The listing builds one solid part. Answer for the finished solid, in the listing's coordinates (mm). A direction names the side the tool comes from. Coordinates: 2 decimals unless noted, no trailing zeros. Order: outer loops, then holes, each group sorted by start corner. A loop starts at its lowest first (then second) coordinate and runs counter-clockwise, first axis right, second up. Notation, with made-up numbers: (-31, 64.5) -> (3, 64.5) arc R26 ccw to (3, 90.5) -> close; hole circle Ø11 at (43, -30). An arc over 180 degrees is marked (long way). Write each question's results on one line, items separated by ' | '. Start each with the question number.
(1) The part is cut by section B-B, the plane z = 37.5. Give the vertices of the cut face in (x, y), then the cut area to 3 significant figures.
(2) Straight lines are drawn through the part: L1, parallel to Z at x = 0, y = -3.2; L2, parallel to Y at x = -11, z = 35.5; L3, parallel to Z at x = -9.5, y = -5. For each, find the intervals that lie inside material, in ascending order.
(3) Determine the mould class of faces 1 (the face through (0, 0, 12)), 2 (the face through (1.3, -7.8, 2)), 3 (the face through (-13.296, -1.972, 15.154)), 4 (the face through (7, -4, 15)) for opening direction Y: +Y half, -Y half, draft (parallel to the pull), parting line (faces both ways), or undercut.
(4) The part is cut by section C-C, the plane y = -2.75. Give the vertices of the cut face in (x, z), then the cut area to 3 significant figures.
(5) A tool of negligible diameter and unlimited length cuts with its end or side. For faces 5 (the face through (1.2, -10.3, 2)), 6 (the face through (10, -4, 2)), 7 (the face through (-2, -8, 4)), 8 (the face through (0, -5, 0)), 9 (the face through (-10, -4, 2)), from which of +Z, -Z, +X, -X, +Y, -Y can it reach the whole face along a straight path? Write none if from no direction.
(6) The part is cut by section A-A, the plane y = -7.5. Give the vertices of the cut face in (x, z), then the cut area to 3 significant figures.
(7) The part is cut by section D-D, the plane x = -5.5. Give the vertices of the cut face in (y, z), then the cut area to 3 significant figures.
(8) Given pin 1 (8 mm diameter, centred on x = -3, y = -10, fed in from +Z); pin 2 (8 mm diameter, centred on y = -9, z = 21.5, fed in from -X); pin 3 (2 mm diameter, centred on y = -5, z = 2, fed in from +X); pin 4 (3 mm diameter, centred on y = -6, z = 2, fed in from -X), each flat-ended and moving along its own axis, determine where each tip first touches the part or whether it passes through.
```python
from build123d import *

# Parameters (mm, degrees)
F1_DEPTH = 14
F0_R     = 12.5
F2_DEPTH = 4
F3_R     = 5
F5_DEPTH = 4


with BuildPart() as f1:
    # F0 (on Front) → F1 (new body)
    with BuildSketch(Plane.XZ):
        Polygon((-10, 0), (0, 0), (10, 0), (10, 4), (-10, 4), align=None)
    extrude(amount=F1_DEPTH)

    # F0 (on Front) → F2 (join)
    with BuildSketch(Plane.XZ):
        with BuildLine():
            Line((-16.5, 26), (-10, 4))
            Line((-10, 4), (10, 4))
            Line((10, 4), (16.5, 26))
            ThreePointArc((16.5, 26), (0, 42.5), (-16.5, 26))
        make_face()
        with Locations((0, 26)):
            Circle(F0_R, mode=Mode.SUBTRACT)
    extrude(amount=F2_DEPTH)

    # F3
    f3_edges = [f1.edges().sort_by_distance(p)[0] for p in [
        (-10, -14, 2),
        (10, -14, 2),
    ]]
    fillet(f3_edges, radius=F3_R)

    # F4 (on face) → F5 (cut)
    with BuildSketch(Plane.XY.offset(4)):
        Polygon((-2.5, -9), (0, -9), (0, -6.5), align=None)
        Polygon((0, -6.5), (0, -9), (2.5, -9), align=None)
        Polygon((2.5, -9), (0, -9), (0, -11.5), align=None)
        Polygon((0, -11.5), (0, -9), (-2.5, -9), align=None)
    extrude(amount=-F5_DEPTH, mode=Mode.SUBTRACT)


solid = f1.part
```
Established:
1) outline: (-11.83, -4) -> (-4.9, -4) -> (-4.9, 0) -> (-11.83, 0) -> close; (4.9, -4) -> (11.83, -4) -> (11.83, 0) -> (4.9, 0) -> close | area: 55.5 mm^2
2) L1: z = 0 to 13.5, 38.5 to 42.5 | L2: y = -4 to 0 | L3: z = 0 to 4
3) face 1: +Y half | face 2: undercut | face 3: draft | face 4: -Y half
4) outline: (-16.5, 26) -> (-10, 4) -> (-10, 0) -> (10, 0) -> (10, 4) -> (16.5, 26) arc R16.5 ccw to start; hole circle Ø25 at (0, 26) | area: 600 mm^2
5) face 5: +Z, -Z | face 6: -Z, +X, +Y, -Y | face 7: +Z, +X, -X, -Y | face 8: -Z, +X, -X, +Y, -Y | face 9: -Z, -X, +Y, -Y
6) outline: (-10, 0) -> (-1, 0) -> (-1, 4) -> (-10, 4) -> close; (1, 0) -> (10, 0) -> (10, 4) -> (1, 4) -> close | area: 72.0 mm^2
7) outline: (-13.97, 0) -> (0, 0) -> (0, 14.78) -> (-4, 14.78) -> (-4, 4) -> (-13.97, 4) -> close; (-4, 37.22) -> (0, 37.22) -> (0, 41.56) -> (-4, 41.56) -> close | area: 116 mm^2
8) pin 1: stops at z = 4 | pin 2: passes through | pin 3: stops at x = 10 | pin 4: stops at x = -10
